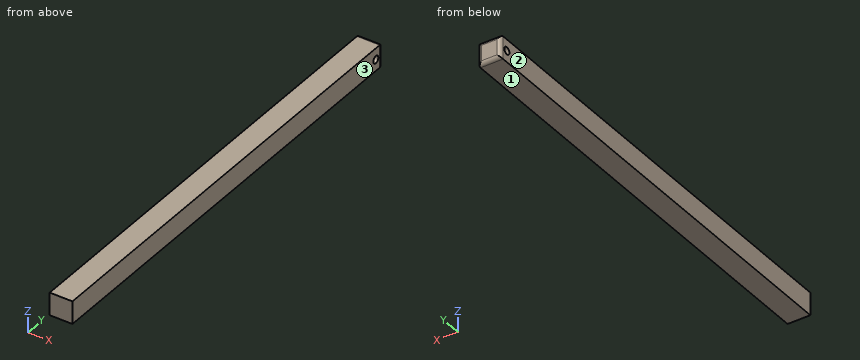
from build123d import *

# Parameters (mm, degrees)
CUT_EXTRUDE1_DEPTH      = 258.20505856
CUT_EXTRUDE1_DEPTH_BACK = 258.20505856
SKETCH2_R               = 4
FILLET1_R               = 4
SCALE1_SCALE            = 5


with BuildPart() as part:
    # Sweep1: sweep along a path in Sketch1
    with BuildLine(Plane.XY) as sweep1_path:
        Line((0, 244.318181818), (0, -255.681818182))
    # 3DSketch1 → Sweep1 (sweep)
    with BuildSketch(Plane(origin=(12.5, -255.681818182, -12.5), x_dir=(-0.7071067811865476, 0, 0.7071067811865476), z_dir=(0, 1, 0))):
        Polygon((0, 0), (17.67766953, 17.67766953), (35.355339059, 0), (17.67766953, -17.67766953), align=None)
    sweep(path=sweep1_path.line)

    # Sketch2 → Cut-Extrude1 (cut, two sides: drawn at the far end of the back side and taken through both)
    with BuildSketch(Plane(origin=(12.5, 0, 0), x_dir=(0, 0, -1), z_dir=(1, 0, 0)).offset(-CUT_EXTRUDE1_DEPTH_BACK)):
        with Locations((0, 234.318181818)):
            Circle(SKETCH2_R)
    extrude(amount=CUT_EXTRUDE1_DEPTH + CUT_EXTRUDE1_DEPTH_BACK, mode=Mode.SUBTRACT)

    # Fillet1
    fillet1_edges = [part.edges().sort_by_distance(p)[0] for p in [
        (-12.5, 244.318181818, 0),
        (0, 244.318181818, -12.5),
        (12.5, 244.318181818, 0),
        (0, 244.318181818, 12.5),
    ]]
    fillet(fillet1_edges, radius=FILLET1_R)


with BuildPart() as part_1:
    # Scale1: scaled about (0, 0, 0)
    add(part.part.scale(SCALE1_SCALE))


solid = part_1.part
Can you work these out from the model? Positions are in its coordinate system, mm. Face numbers are marked on the shaded views. Coordinates: 2 decimals unless noted, no trailing zeros. Loops run counter-clockwise (first coordinate to the right, second up) from the corner with the lowest first, then second, coordinate; pieces in that order, holes last. Notation, with made-up numbers: (26.25, -15.75) - (84.25, -15.75) arc R21 ccw to (84.25, -8.75) - close; hole circle Ø7 at (-8, 15.25). An arc over 180 degrees is marked (long way). Put each result on its own line as item: value. Start each with the question number.
Item 1: If we mould it in two halves opening along X, with no side actions, what happens to the marked faces 1, 2 and 3? For each: +X half, -X half, draft (parallel to the pull), parting line (faces both ways), or undercut.
Item 2: Suppose I cut it at A-A (z = 0). Please give me the cut outline in (x, y), and give its area (3 significant figures).
Item 3: If I drill on line 1 along Y through (x, z) = (28, 0); line 2 along Y through (x, z) = (-11.5, 13); line 3 along Y through (x, z) = (-15.5, 47.5), over which ranges is the centre line in solid material (lowest first)?
Here are the results:
1. face 1: draft
1. face 2: -X half
1. face 3: +X half
2. outline: (-62.5, -1278.41) - (62.5, -1278.41) - (62.5, 1151.59) - (-62.5, 1151.59) - close; (-62.5, 1191.59) - (62.5, 1191.59) - (62.5, 1201.59) arc R20 ccw to (42.5, 1221.59) - (-42.5, 1221.59) arc R20 ccw to (-62.5, 1201.59) - close
2. area: 307,000 mm²
3. line 1: -1278.41 to 1151.59, 1191.59 to 1221.59
3. line 2: -1278.41 to 1156.39, 1186.79 to 1221.59
3. line 3: -1278.41 to 1220.96
